```python
from build123d import *

# Parameters (mm, degrees)
SKETCH1_W                = 158
SKETCH1_H                = 199.5
BOSS_EXTRUDE1_DEPTH      = 6.35
SKETCH2_W                = 81
SKETCH2_H                = 41
CUT_EXTRUDE1_DEPTH       = 7.35
BOSS_EXTRUDE2_DEPTH      = 12.7
M4_CLEARANCE_HOLE1_D     = 4.5
M4_CLEARANCE_HOLE1_DEPTH = 6.35
CUT_EXTRUDE2_REACH       = 201.5
SKETCH7_W                = 129
SKETCH7_H                = 10
FILLET1_R                = 5
M4_CLEARANCE_HOLE2_D     = 4.5
M4_CLEARANCE_HOLE2_DEPTH = 6.35
LPATTERN1_COUNT          = 4
LPATTERN1_PITCH          = 30
LPATTERN1_COUNT_DIR2     = 3
LPATTERN1_PITCH_DIR2     = 37.5


with BuildPart() as part:
    # Sketch1 → Boss-Extrude1 (new body)
    with BuildSketch(Plane(origin=(0, 0, 0), x_dir=(1, 0, 0), z_dir=(0, 1, 0))):
        with Locations((79, -99.75)):
            Rectangle(SKETCH1_W, SKETCH1_H)
    extrude(amount=BOSS_EXTRUDE1_DEPTH)

    # Sketch2 → Cut-Extrude1 (cut, through all)
    with BuildSketch(Plane(origin=(0, 6.35, 0), x_dir=(1, 0, 0), z_dir=(0, 1, 0))):
        with Locations((40.5, -179)):
            Rectangle(SKETCH2_W, SKETCH2_H)
    extrude(amount=-CUT_EXTRUDE1_DEPTH, mode=Mode.SUBTRACT)

    # Sketch3 → Boss-Extrude2 (add)
    with BuildSketch(Plane(origin=(0, 6.35, 0), x_dir=(1, 0, 0), z_dir=(0, 1, 0))):
        Polygon((158, 0), (158, -5), (5, -5), (5, -153.5), (86, -153.5), (86, -194.5), (158, -194.5), (158, -199.5), (86, -199.5), (81, -199.5), (81, -158.5), (0, -158.5), (0, 0), align=None)
    extrude(amount=BOSS_EXTRUDE2_DEPTH)

    # M4 Clearance Hole1
    with Locations(Plane.XZ):
        with Locations((20, 54.25), (99.5, 179.5), (139.5, 179.5), (20, 129.25), (20, 104.25), (20, 29.25)):
            Hole(M4_CLEARANCE_HOLE1_D / 2, depth=M4_CLEARANCE_HOLE1_DEPTH)

    # Sketch7 → Cut-Extrude2 (cut, up to next)
    with BuildSketch(Plane(origin=(0, 0, 0), x_dir=(-1, 0, 0), z_dir=(0, 0, -1)), mode=Mode.PRIVATE) as cut_extrude2_sk1:
        with Locations((-93.5, 14.05)):
            Rectangle(SKETCH7_W, SKETCH7_H)
    cut_extrude2_tool1 = extrude(cut_extrude2_sk1.sketch, amount=-CUT_EXTRUDE2_REACH, mode=Mode.PRIVATE) & part.part
    add(cut_extrude2_tool1.solids().sort_by_distance((93.5, 14.05, 0))[0], mode=Mode.SUBTRACT)

    # Fillet1
    fillet1_edges = [part.edges().sort_by_distance(p)[0] for p in [
        (29, 9.05, 2.5),
    ]]
    fillet(fillet1_edges, radius=FILLET1_R)

    # M4 Clearance Hole2
    with Locations(Plane(origin=(0, 6.35, 0), x_dir=(1, 0, 0), z_dir=(0, 1, 0))):
        with Locations((138, -116.75)):
            m4_clearance_hole2 = Hole(M4_CLEARANCE_HOLE2_D / 2, depth=M4_CLEARANCE_HOLE2_DEPTH)

    # LPattern1: M4 Clearance Hole2 4 × 3
    with Locations(*[(-i * LPATTERN1_PITCH, 0, -j * LPATTERN1_PITCH_DIR2) for i in range(LPATTERN1_COUNT) for j in range(LPATTERN1_COUNT_DIR2) if (i, j) != (0, 0)]):
        add(m4_clearance_hole2, mode=Mode.SUBTRACT)


solid = part.part
```
Geometry: final body of the model. Coordinates: model frame, mm. A direction names the side the tool comes from. Give positions to 0.01 mm unless a question says otherwise; leave off trailing zeros. Write each loop counter-clockwise with the first axis right and the second up, starting at its lowest first coordinate (ties: lowest second). Pieces come first, ordered by that corner, then holes.
1. Draft query along X for faces 4 (the cylindrical face through (30.5, 10.48, 2.54)), 5 (the cylindrical face through (48, 3, 119)), 6 (the flat face through (97, 9.05, 2)). Return one class per face: released by +X, released by -X, zero draft, split by the parting line, or undercut.
2. Section query C-C, the plane x = 20. Return loops of the section in (y, z), then the cut area to 3 significant figures.
3. Section query B-B, the plane z = 41.75. Return loops of the section in (x, y).
4. Section query A-A, the plane x = 99.5. Return loops of the section in (y, z), then the cut area to 3 significant figures.
5. Pin query (flat end, axial travel): P1, Ø6, axis at x = 62.5, y = 12.5, coming from the -Z side; P2, Ø4, axis at x = 108, z = 41.75, coming from the +Y side; P3, Ø4, axis at y = 17, z = 2.5, coming from the +X side; P4, Ø4, axis at y = 9.5, z = 58, coming from the +X side. Return the tip coordinate at first contact, or that it passes through.
6. Line query: probe 1 along Z at (x, y) = (78, 4); probe 2 along X at (y, z) = (3, 116.75); probe 3 along X at (y, z) = (3.25, 179.5). Output: solid intervals per line, ascending.
7. Section query D-D, the plane z = 179.5. Return loops of the section in (x, y), then the cut area to 3 significant figures.
8. Reachability of faces 1 (the flat face through (119, 9, 199.5)), 2 (the flat face through (29, 17, 2)), 3 (the flat face through (41, 9, 158.5)) from +Z, -Z, +X, -X, +Y, -Y: full face, straight path, thin tool, end or side. Return the list, or none.
Computed:
1. face 4: released by +X
1. face 5: undercut
1. face 6: zero draft
2. outline: (0, 0) - (19.05, 0) - (19.05, 5) - (6.35, 5) - (6.35, 27) - (0, 27) - close; (0, 31.5) - (6.35, 31.5) - (6.35, 52) - (0, 52) - close; (0, 56.5) - (6.35, 56.5) - (6.35, 102) - (0, 102) - close; (0, 106.5) - (6.35, 106.5) - (6.35, 127) - (0, 127) - close; (0, 131.5) - (6.35, 131.5) - (6.35, 153.5) - (19.05, 153.5) - (19.05, 158.5) - (0, 158.5) - close
2. area: 1,020 mm2
3. outline: (0, 0) - (45.75, 0) - (45.75, 6.35) - (5, 6.35) - (5, 19.05) - (0, 19.05) - close; (50.25, 0) - (75.75, 0) - (75.75, 6.35) - (50.25, 6.35) - close; (80.25, 0) - (105.75, 0) - (105.75, 6.35) - (80.25, 6.35) - close; (110.25, 0) - (135.75, 0) - (135.75, 6.35) - (110.25, 6.35) - close; (140.25, 0) - (158, 0) - (158, 6.35) - (140.25, 6.35) - close
4. outline: (0, 0) - (9.05, 0) - (9.05, 5) - (6.35, 5) - (6.35, 177.25) - (0, 177.25) - close; (0, 181.75) - (6.35, 181.75) - (6.35, 194.5) - (19.05, 194.5) - (19.05, 199.5) - (0, 199.5) - close
4. area: 1,320 mm2
5. P1: stops at z = 153.5
5. P2: passes through
5. P3: stops at x = 29
5. P4: stops at x = 5
6. probe 1: z = 0 to 39.5, 44 to 77, 81.5 to 114.5, 119 to 158.5
6. probe 2: x = 0 to 45.75, 50.25 to 75.75, 80.25 to 105.75, 110.25 to 135.75, 140.25 to 158
6. probe 3: x = 81 to 97.25, 101.75 to 137.25, 141.75 to 158
7. outline: (81, 0) - (97.25, 0) - (97.25, 6.35) - (86, 6.35) - (86, 19.05) - (81, 19.05) - close; (101.75, 0) - (137.25, 0) - (137.25, 6.35) - (101.75, 6.35) - close; (141.75, 0) - (158, 0) - (158, 6.35) - (141.75, 6.35) - close
7. area: 495 mm2
8. face 1: +Z, +X, -X, +Y, -Y
8. face 2: -Z, +X, +Y
8. face 3: +Z, -X, +Y, -Y
